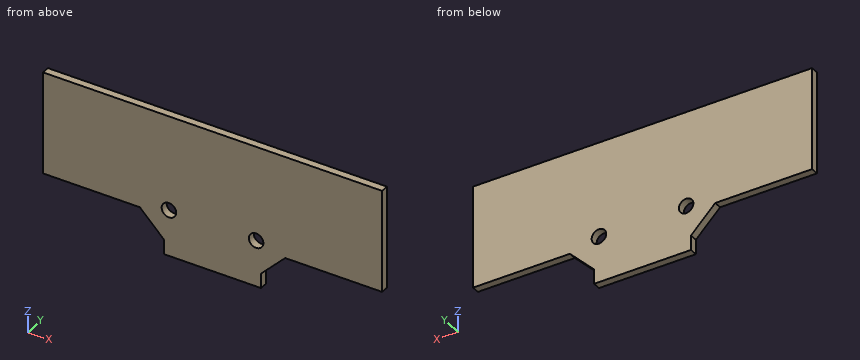
```python
from build123d import *

# Parameters (mm, degrees)
SKETCH_1_R      = 1.5
EXTRUDE_1_DEPTH = 1.6


with BuildPart() as part:
    # 草图1 → 凸台-拉伸1 (new body)
    with BuildSketch(Plane(origin=(0, 0, 0), x_dir=(1, 0, 0), z_dir=(0, 1, 0))):
        Polygon((-9.701583435, 20.645554202), (-14.701583435, 15.645554202), (-34.701583435, 15.645554202), (-34.701583435, -5.354445798), (35.298416565, -5.354445798), (35.298416565, 15.645554202), (15.298416565, 15.645554202), (10.298416565, 20.645554202), (10.298416565, 23.645554202), (-9.701583435, 23.645554202), align=None)
        with Locations(Location((-8.701583435, 14.145554202, 0), (0, 0, 270))):
            Circle(SKETCH_1_R, mode=Mode.SUBTRACT)
        with Locations(Location((9.298416565, 14.145554202, 0), (0, 0, 270))):
            Circle(SKETCH_1_R, mode=Mode.SUBTRACT)
    extrude(amount=EXTRUDE_1_DEPTH)


solid = part.part
```
Geometry check sheet. Reference: the model listing, model coordinates, mm. Give positions to 0.01 mm unless a question says otherwise; leave off trailing zeros. Order: outer loops, then holes, each group sorted by start corner. A loop starts at its lowest first (then second) coordinate and runs counter-clockwise, first axis right, second up. Notation, with made-up numbers: (41, 24.5) - (100, 24.5) arc R16 cw to (100, 43.5) - close; hole circle Ø6 at (57.25, -2.75). An arc over 180 degrees is marked (long way). Answer in a Markdown table with one row per item. Add a question column.
Q1. Cross-section at A-A, the plane y = 0.8. Enter the section's corners in (x, z), then the cut area to 3 significant figures.
Q2. Material ranges on probe 1 along X at (y, z) = (1.25, -13.75); probe 2 along X at (y, z) = (0.5, -15); probe 3 along Z at (x, y) = (32, 1.4), recorded low to high. Write a range as from..to.
Q3. Gauge pin test, flat end, axial feed: pin 1 (0.8 mm diameter, centred on x = -24, y = 1, fed in from -Z). Record the tip position at first contact, or that the pin passes through.
Q4. Cross-section at C-C, the plane z = -21.5. Enter the section's corners in (x, y), then the cut area to 3 significant figures.
Q5. Cross-section at B-B, the plane x = -21. Enter the section's corners in (y, z), then the cut area to 3 significant figures.
Check values:
| question | item | result |
|---|---|---|
| 1 | outline | (-34.7, -15.65) - (-14.7, -15.65) - (-9.7, -20.65) - (-9.7, -23.65) - (10.3, -23.65) - (10.3, -20.65) - (15.3, -15.65) - (35.3, -15.65) - (35.3, 5.35) - (-34.7, 5.35) - close; hole circle Ø3 at (-8.7, -14.15); hole circle Ø3 at (9.3, -14.15) |
| 1 | area | 1,640 mm^2 |
| 2 | probe 1 | x = -34.7..-10.15, -7.25..7.85, 10.75..35.3 |
| 2 | probe 2 | x = -34.7..-9.93, -7.47..8.07, 10.53..35.3 |
| 2 | probe 3 | z = -15.65..5.35 |
| 3 | pin 1 | stops at z = -15.65 |
| 4 | outline | (-9.7, 0) - (10.3, 0) - (10.3, 1.6) - (-9.7, 1.6) - close |
| 4 | area | 32.0 mm^2 |
| 5 | outline | (0, -15.65) - (1.6, -15.65) - (1.6, 5.35) - (0, 5.35) - close |
| 5 | area | 33.6 mm^2 |
